from build123d import *

# Parameters (mm, degrees)
SKETCH_W           = 43
SKETCH_H           = 180
SKETCH_W_2         = 75.5
SKETCH_H_2         = 43
SKETCH_W_3         = 36
SKETCH_H_3         = 36.5
PAD_DEPTH          = 15
SKETCH002_W        = 100
SKETCH002_H        = 5
SKETCH002_W_2      = 5
SKETCH002_H_2      = 107
PAD001_DEPTH       = 10
SKETCH003_W        = 5
SKETCH003_H        = 93
SKETCH003_W_2      = 86
SKETCH003_H_2      = 5
PAD002_DEPTH       = 15
SKETCH004_R        = 2.6
POCKET_DEPTH       = 138.5
SKETCH005_R        = 5.5
POCKET001_DEPTH    = 88.5
POCKET005_START    = -1.875
POCKET005_DEPTH    = 3.25
SKETCH010_R        = 4.5
POCKET006_DEPTH    = 3.3
CHAMFER001_1_SIZE2 = 3
CHAMFER001_1_SIZE  = 1.75
CHAMFER001_2_SIZE2 = 3
CHAMFER001_2_SIZE  = 1.75
SKETCH014_R        = 2.6
POCKET008_DEPTH    = 20
POCKET011_START    = -3.75
POCKET011_DEPTH    = 3.5
POCKET012_START    = -3.75
POCKET012_DEPTH    = 3.5


with BuildPart() as part:
    # Sketch → Pad (new body)
    with BuildSketch(Plane.XY):
        Polygon((124, 0), (124, 180), (124, 186), (24, 186), (24, 180), (24, 143.5), (-8.5, 143.5), (-14.5, 143.5), (-14.5, 36.5), (-8.5, 36.5), (24, 36.5), (24, 0), (24, -6), (124, -6), align=None)
        with Locations((95.5, 90)):
            Rectangle(SKETCH_W, SKETCH_H, mode=Mode.SUBTRACT)
        with Locations((29.25, 115)):
            Rectangle(SKETCH_W_2, SKETCH_H_2, mode=Mode.SUBTRACT)
        with Locations((29.25, 65)):
            Rectangle(SKETCH_W_2, SKETCH_H_2, mode=Mode.SUBTRACT)
        with Locations((49, 161.75)):
            Rectangle(SKETCH_W_3, SKETCH_H_3, mode=Mode.SUBTRACT)
        with Locations((49, 18.25)):
            Rectangle(SKETCH_W_3, SKETCH_H_3, mode=Mode.SUBTRACT)
    extrude(amount=PAD_DEPTH)

    # Sketch002 (on Face25 of Pad) → Pad001 (join)
    with BuildSketch(Plane.XY.offset(15)):
        with Locations((74, 183.5)):
            Rectangle(SKETCH002_W, SKETCH002_H)
        with Locations((74, -3.5)):
            Rectangle(SKETCH002_W, SKETCH002_H)
        with Locations((-12, 90)):
            Rectangle(SKETCH002_W_2, SKETCH002_H_2)
    extrude(amount=PAD001_DEPTH)

    # Sketch003 (on Face4 of Pad001) → Pad002 (join)
    with BuildSketch(Plane(origin=(0, 0, 0), x_dir=(1, 0, 0), z_dir=(0, 0, -1))):
        with Locations((-6, -90)):
            Rectangle(SKETCH003_W, SKETCH003_H)
        with Locations((74, -177.5)):
            Rectangle(SKETCH003_W_2, SKETCH003_H_2)
        with Locations((74, -2.5)):
            Rectangle(SKETCH003_W_2, SKETCH003_H_2)
    extrude(amount=-PAD002_DEPTH)

    # Sketch004 (on Face35 of Pad002) → Pocket (cut)
    with BuildSketch(Plane(origin=(-14.5, 0, 0), x_dir=(0, -1, 0), z_dir=(-1, 0, 0))):
        with Locations((-115, 7.5)):
            Circle(SKETCH004_R)
        with Locations((-20.75, 7.5)):
            Circle(SKETCH004_R)
        with Locations((-65, 7.5)):
            Circle(SKETCH004_R)
        with Locations((-159.25, 7.5)):
            Circle(SKETCH004_R)
    extrude(amount=-POCKET_DEPTH, mode=Mode.SUBTRACT)

    # Sketch005 (on Face17 of Pocket) → Pocket001 (cut)
    with BuildSketch(Plane(origin=(-14.5, 0, 0), x_dir=(0, -1, 0), z_dir=(-1, 0, 0))):
        with Locations((-159.25, 7.5)):
            Circle(SKETCH005_R)
        with Locations((-20.75, 7.5)):
            Circle(SKETCH005_R)
    extrude(amount=-POCKET001_DEPTH, mode=Mode.SUBTRACT)

    # Sketch009 (on Face3 of Pocket001) → Pocket005 (cut)
    with BuildSketch(Plane.YZ.offset(124).offset(POCKET005_START)):
        Polygon((60.275, 10.22798), (60.275, 4.77202), (65, 2.04404), (69.725, 4.77202), (69.725, 10.22798), (69.725, 15), (60.275, 15), align=None)
        Polygon((110.275, 10.22798), (110.275, 4.77202), (115, 2.04404), (119.725, 4.77202), (119.725, 10.22798), (119.725, 15), (110.275, 15), align=None)
    extrude(amount=-POCKET005_DEPTH, mode=Mode.SUBTRACT)

    # Sketch010 (on Face21 of Pocket005) → Pocket006 (cut)
    with BuildSketch(Plane(origin=(117, 0, 0), x_dir=(0, -1, 0), z_dir=(-1, 0, 0))):
        with Locations((-159.25, 7.5)):
            Circle(SKETCH010_R)
        with Locations((-20.75, 7.5)):
            Circle(SKETCH010_R)
    extrude(amount=-POCKET006_DEPTH, mode=Mode.SUBTRACT)

    # Chamfer001 1
    chamfer001_1_edges = [part.edges().sort_by_distance(p)[0] for p in [
        (120.3, 163.75, 7.5),
    ]]
    chamfer001_1_side = part.faces().sort_by_distance((120.3, 163.622721, 7.5))[0]
    chamfer(chamfer001_1_edges, length=CHAMFER001_1_SIZE, length2=CHAMFER001_1_SIZE2, reference=chamfer001_1_side)

    # Chamfer001 2
    chamfer001_2_edges = [part.edges().sort_by_distance(p)[0] for p in [
        (120.3, 25.25, 7.5),
    ]]
    chamfer001_2_side = part.faces().sort_by_distance((120.3, 25.122721, 7.5))[0]
    chamfer(chamfer001_2_edges, length=CHAMFER001_2_SIZE, length2=CHAMFER001_2_SIZE2, reference=chamfer001_2_side)

    # Sketch014 (on Face10 of Chamfer001) → Pocket008 (cut)
    with BuildSketch(Plane(origin=(0, 186, 0), x_dir=(-1, 0, 0), z_dir=(0, 1, 0))):
        with Locations((-99, 7.5)):
            Circle(SKETCH014_R)
    extrude(amount=-POCKET008_DEPTH, mode=Mode.SUBTRACT)

    # Sketch018 (on Face25 of Pocket008) → Pocket011 (cut)
    with BuildSketch(Plane(origin=(-14.5, 0, 0), x_dir=(0, -1, 0), z_dir=(-1, 0, 0)).offset(POCKET011_START)):
        Polygon((-115, 12.95596), (-119.725, 10.22798), (-119.725, 4.77202), (-119.725, 0), (-110.275, 0), (-110.275, 4.77202), (-110.275, 10.22798), align=None)
        Polygon((-69.725, 10.22798), (-69.725, 4.77202), (-69.725, 0), (-60.275, 0), (-60.275, 4.77202), (-60.275, 10.22798), (-65, 12.95596), align=None)
    extrude(amount=-POCKET011_DEPTH, mode=Mode.SUBTRACT)

    # Sketch019 (on Face10 of Pocket011) → Pocket012 (cut)
    with BuildSketch(Plane(origin=(0, 186, 0), x_dir=(-1, 0, 0), z_dir=(0, 1, 0)).offset(POCKET012_START)):
        Polygon((-94.275, 10.22798), (-99, 12.95596), (-103.725, 10.22798), (-103.725, 4.77202), (-103.725, 0), (-94.275, 0), (-94.275, 4.77202), align=None)
    extrude(amount=-POCKET012_DEPTH, mode=Mode.SUBTRACT)


solid = part.part
Work out the finished part from the listing and answer in its coordinate system (mm). A direction names the side the tool comes from. Give positions to 0.01 mm unless a question says otherwise; leave off trailing zeros. Write each loop counter-clockwise with the first axis right and the second up, starting at its lowest first coordinate (ties: lowest second). Pieces come first, ordered by that corner, then holes. Notation, with made-up numbers: M -30,-3 L -23,-3 A10 cw -23,2 Z; hole C 59,33 d4. An arc over 180 degrees is marked long. Answer as CSV lines item,"result".
Q1. A tool of negligible diameter and unlimited length cuts with its end or side. For faces 4 (the flat face through (73, 181, 20)), 5 (the cylindrical face through (70.45, 18.21, 2.62)), 6 (the cylindrical face through (101.6, 176.9, 7.6)), from which of +Z, -Z, +X, -X, +Y, -Y can it reach the whole face along a straight path? Write none if from no direction.
A:
face 4,"+Z, +X, -X"
face 5,"-X"
face 6,"+Y"
Q2. A cutting plane is placed at A-A on x = 48. Write down the section's boundary in (y, z), plus the area to 3 significant figures.
A:
outline,"M -6,0 L 5,0 L 5,15 L -1,15 L -1,25 L -6,25 Z; M 36.5,0 L 43.5,0 L 43.5,15 L 36.5,15 Z; M 86.5,0 L 93.5,0 L 93.5,15 L 86.5,15 Z; M 136.5,0 L 143.5,0 L 143.5,15 L 136.5,15 Z; M 175,0 L 186,0 L 186,25 L 181,25 L 181,15 L 175,15 Z"
area,"745 mm²"
Q3. A cutting plane is placed at C-C on y = 149.5. Write down the section's boundary in (x, z), plus the area to 3 significant figures.
A:
outline,"M 24,0 L 31,0 L 31,15 L 24,15 Z; M 67,0 L 74,0 L 74,15 L 67,15 Z; M 117,0 L 124,0 L 124,15 L 117,15 Z"
area,"315 mm²"
Q4. A cutting plane is placed at B-B on z = 20. Write down the section's boundary in (x, y).
A:
outline,"M -14.5,36.5 L -9.5,36.5 L -9.5,143.5 L -14.5,143.5 Z; M 24,-6 L 124,-6 L 124,-1 L 24,-1 Z; M 24,181 L 124,181 L 124,186 L 24,186 Z"
Q5. Find the intervals of material crossed by probe 1 along X at (y, z) = (150.5, 8); probe 2 along X at (y, z) = (60.5, 6.25) (3 decimals); probe 3 along Y at (x, z) = (103, 6.75), in increasing order. Write a range as [from, to].
A:
probe 1,"x = [24, 31], [67, 74], [117, 124]"
probe 2,"x = [-14.5, -10.75], [-7.25, -3.5], [67, 74], [117, 118.875], [122.125, 124]"
probe 3,"y = [-6, 5], [175, 178.75], [182.25, 186]"
Q6. A cutting plane is placed at D-D on y = 20.75. Count the separate pieces of the cut face and the enclosed holes in it, plus the area to 3 significant figures.
A:
separate pieces,"6"
enclosed holes,"0"
area,"117 mm²"
Q7. Given P1, Ø3, axis at x = -8, z = 6, coming from the -Y side; P2, Ø5, axis at y = 166, z = 10.5, coming from the -X side; P3, Ø12.5, axis at x = 6, z = 10, coming from the +Y side, each flat-ended and moving along its own axis, determine where each tip first touches the part or whether it passes through.
A:
P1,"stops at y = 36.5"
P2,"stops at x = 24"
P3,"stops at y = 143.5"
Q8. The mould has two halves that part along Z. Classify faces 1 (the flat face through (31, 93.5, 7)), 2 (the flat face through (73, -3, 25)), 3 (the cylindrical face through (101.6, 184.2, 7.6)): +Z half, -Z half, draft (parallel to the pull), parting line (faces both ways), or undercut.
A:
face 1,"draft"
face 2,"+Z half"
face 3,"undercut"
